Autodesk Inventor part; units mm, degrees
ref_plane "YZ Plane" through (0, 0, 0) normal (1, 0, 0) x (0, 1, 0)
ref_plane "XZ Plane" through (0, 0, 0) normal (0, 1, 0) x (-1, 0, 0)
ref_plane "XY Plane" through (0, 0, 0) normal (0, 0, 1) x (1, 0, 0)
sketch "スケッチ1" plane through (0, 0, 0) normal (0, 1, 0) x (-1, 0, 0)
  arc A0 (0, -8) -> (4.5997, -6.5455) centre (0, 0) ccw
  line L0 (33, -28) -> (33, -20) construction
  line L1 (0, 0) -> (0, -13.0211) construction
  circle A1 centre (33, -28) radius 1.05
  circle A2 centre (33, -20) radius 1.05
  line L2 (31, -31) -> (9.1961, -6.9835)
  line L3 (31, -31) -> (35, -31)
  line L4 (35, -31) -> (35, -17)
  line L5 (35, -17) -> (8.0357, 2.5722)
  line L6 (31, -22.8462) -> (31, -17.5875)
  line L7 (30.1748, -15.969) -> (16.1748, -5.807)
  line L8 (13.5192, -8.7699) -> (27.5192, -24.1906)
  arc A3 (27.5192, -24.1906) -> (31, -22.8462) centre (29, -22.8462) ccw
  arc A4 (31, -17.5875) -> (30.1748, -15.969) centre (29, -17.5875) ccw
  arc A5 (16.1748, -5.807) -> (13.5192, -8.7699) centre (15, -7.4256) ccw
  line L9 (6.9749, -6) -> (6.3246, -6)
  arc A6 (7.1258, 3.6364) -> (0, 8) centre (0, 0) ccw
  line L10 (0, 8) -> (0, 0) construction
  arc A7 (6.3246, -6) -> (4.5997, -6.5455) centre (6.3246, -9) ccw
  arc A8 (7.1258, 3.6364) -> (8.0357, 2.5722) centre (9.798, 5) ccw
  arc A9 (9.1961, -6.9835) -> (6.9749, -6) centre (6.9749, -9) ccw
  arc A10 (-4.5997, -6.5455) -> (0, -8) centre (0, 0) ccw
  line L11 (-33, -28) -> (-33, -20) construction
  circle A11 centre (-33, -28) radius 1.05
  circle A12 centre (-33, -20) radius 1.05
  line L12 (-31, -31) -> (-9.1961, -6.9835)
  line L13 (-31, -31) -> (-35, -31)
  line L14 (-35, -31) -> (-35, -17)
  line L15 (-35, -17) -> (-8.0357, 2.5722)
  line L16 (-31, -22.8462) -> (-31, -17.5875)
  line L17 (-30.1748, -15.969) -> (-16.1748, -5.807)
  line L18 (-13.5192, -8.7699) -> (-27.5192, -24.1906)
  arc A13 (-31, -22.8462) -> (-27.5192, -24.1906) centre (-29, -22.8462) ccw
  arc A14 (-30.1748, -15.969) -> (-31, -17.5875) centre (-29, -17.5875) ccw
  arc A15 (-13.5192, -8.7699) -> (-16.1748, -5.807) centre (-15, -7.4256) ccw
  line L19 (-6.9749, -6) -> (-6.3246, -6)
  arc A16 (0, 8) -> (-7.1258, 3.6364) centre (0, 0) ccw
  arc A17 (-4.5997, -6.5455) -> (-6.3246, -6) centre (-6.3246, -9) ccw
  arc A18 (-8.0357, 2.5722) -> (-7.1258, 3.6364) centre (-9.798, 5) ccw
  arc A19 (-6.9749, -6) -> (-9.1961, -6.9835) centre (-6.9749, -9) ccw
  circle A20 centre (0, 0) radius 4
  point P0 (5.2915, -6)
  point P1 (-5.2915, -6)
  dimension "d0" = 2.1
  dimension "d1" = 8
  dimension "d2" = 4
  dimension "d3" = 3
  dimension "d4" = 3
  dimension "d5" = 70
  dimension "d6" = 2
  dimension "d7" = 2
  dimension "d8" = 2
  dimension "d10" = 8
  dimension "d11" = 3
  dimension "d12" = 20
  dimension "d13" = 6
  dimension "d14" = 5
  dimension "d15" = 15
  dimension "d16" = 8
extrude "押し出し1" add sketch "スケッチ1" along normal blind 2
properties part number "shoulder"
Input: part model. Units: mm. Frame: model coordinates. A direction names the side the tool comes from. Coordinates: 2 decimals unless noted, no trailing zeros. Order: outer loops, then holes, each group sorted by start corner. A loop starts at its lowest first (then second) coordinate and runs counter-clockwise, first axis right, second up. Notation, with made-up numbers: M -35.5,47.25 L -23.5,47.25 A13 ccw -23.5,59.25 Z; hole C -28.5,18.25 d8. An arc over 180 degrees is marked long. Write item = value, one per line. Start each with the question number.
(1) Reachability of faces 1 (the flat face through (-33, 1, -31)), 2 (the flat face through (-20.25, 0.99, -19.16)), 3 (the flat face through (31, 1, -20)) from +Z, -Z, +X, -X, +Y, -Y: full face, straight path, thin tool, end or side. Return the list, or none.
(2) Line query: line 1 along Z through (x, y) = (-33, 0.7); line 2 along X through (y, z) = (1.25, -22); line 3 along Z through (x, y) = (22, 0.2). Output: solid intervals per line, ascending. Write a range as [from, to].
(3) Section C-C on z = -26. Output: boundary loops of the cut face in (x, y).
(4) Section B-B on x = 33. Output: boundary loops of the cut face in (y, z).
(5) Pull-direction query (X, two-part tool) for faces 4 (the flat face through (20.25, 0.99, -19.16)), 5 (the flat face through (21.707, 0.986, -7.351)), 6 (the flat face through (-21.707, 0.986, -7.351)); classes: released by +X, released by -X, zero draft, split by the parting line, or undercut.
(6) Section D-D on x = -20. Output: boundary loops of the cut face in (y, z).
(7) Section A-A on z = -20. Output: boundary loops of the cut face in (x, y).
(8) First-contact query: P1, Ø0.7, axis at x = -6.5, y = 1, coming from the -Z side. Flat tip, straight axial feed; report the tip coordinate or a pass-through.
Result set:
q1.face_1 = -Z, +X, -X, +Y, -Y
q1.face_2 = -Z, +Y, -Y
q1.face_3 = +Y, -Y
q2.line_1 = [-31, -29.05], [-26.95, -21.05], [-18.95, -15.55]
q2.line_2 = [-35, -31], [-25.53, -22.83], [22.83, 25.53], [31, 35]
q2.line_3 = [-21.09, -18.11], [-10.04, -7.56]
q3.outline = M -35,0 L -26.46,0 L -26.46,2 L -35,2 Z; M 26.46,0 L 35,0 L 35,2 L 26.46,2 Z
q4.outline = M 0,-31 L 2,-31 L 2,-29.05 L 0,-29.05 Z; M 0,-26.95 L 2,-26.95 L 2,-21.05 L 0,-21.05 Z; M 0,-18.95 L 2,-18.95 L 2,-15.55 L 0,-15.55 Z
q5.face_4 = undercut
q5.face_5 = released by +X
q5.face_6 = released by -X
q6.outline = M 0,-18.88 L 2,-18.88 L 2,-15.91 L 0,-15.91 Z; M 0,-8.58 L 2,-8.58 L 2,-6.11 L 0,-6.11 Z
q7.outline = M -35,0 L -34.05,0 L -34.05,2 L -35,2 Z; M -31.95,0 L -31,0 L -31,2 L -31.95,2 Z; M -23.71,0 L -21.01,0 L -21.01,2 L -23.71,2 Z; M 21.01,0 L 23.71,0 L 23.71,2 L 21.01,2 Z; M 31,0 L 31.95,0 L 31.95,2 L 31,2 Z; M 34.05,0 L 35,0 L 35,2 L 34.05,2 Z
q8.P1 = -6.01
